from build123d import *

# Parameters (mm, degrees)
SKETCH1_R           = 10
BOSS_EXTRUDE1_DEPTH = 75
SKETCH2_R           = 9.5
CUT_EXTRUDE1_DEPTH  = 77.321687612
SKETCH4_W           = 0.5
SKETCH4_H           = 10


with BuildPart() as part:
    # Sketch1 → Boss-Extrude1 (new body)
    with BuildSketch(Plane(origin=(0, 0, 0), x_dir=(1, 0, 0), z_dir=(0, 1, 0))):
        with Locations(Location((0, 0, 0), (0, 0, 270))):
            Circle(SKETCH1_R)
    extrude(amount=BOSS_EXTRUDE1_DEPTH)

    # Sketch2 → Cut-Extrude1 (cut, through all)
    with BuildSketch(Plane(origin=(0, 75, 0), x_dir=(1, 0, 0), z_dir=(0, 1, 0))):
        with Locations(Location((0, 0, 0), (0, 0, 270))):
            Circle(SKETCH2_R)
    extrude(amount=-CUT_EXTRUDE1_DEPTH, mode=Mode.SUBTRACT)

    # Sketch3 → Revolve1 (revolve)
    with BuildSketch(Plane(origin=(0, 0, 0), x_dir=(0, 0, -1), z_dir=(1, 0, 0)), mode=Mode.PRIVATE) as revolve1_sk:
        Polygon((10, 75), (12.75, 85), (12.25, 85), (9.5, 75), align=None)
    revolve(revolve1_sk.sketch.rotate(Axis((0, 75, 0), (0, -1, 0)), 180), axis=Axis((0, 75, 0), (0, -1, 0)))

    # Sketch4 → Revolve2 (revolve)
    with BuildSketch(Plane(origin=(0, 0, 0), x_dir=(0, 0, -1), z_dir=(1, 0, 0)), mode=Mode.PRIVATE) as revolve2_sk:
        with Locations((12.5, 90)):
            Rectangle(SKETCH4_W, SKETCH4_H)
    revolve(revolve2_sk.sketch.rotate(Axis((0, 75, 0), (0, -1, 0)), 180), axis=Axis((0, 75, 0), (0, -1, 0)))


solid = part.part
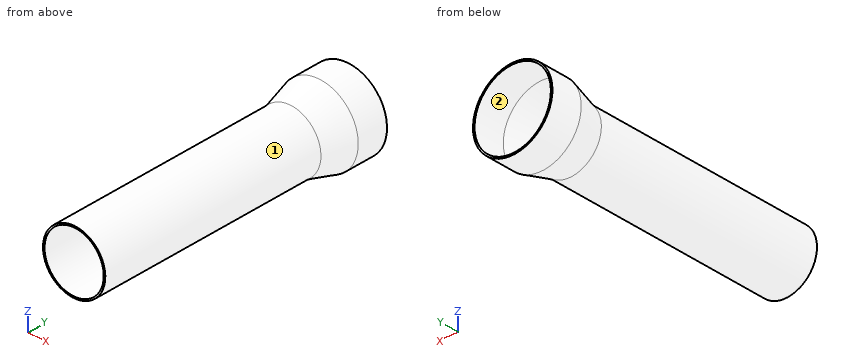
Can you work these out from the model? Positions are in its coordinate system, mm. Face numbers are marked on the shaded views. Give positions to 0.01 mm unless a question says otherwise; leave off trailing zeros. Order: outer loops, then holes, each group sorted by start corner. A loop starts at its lowest first (then second) coordinate and runs counter-clockwise, first axis right, second up. Notation, with made-up numbers: M 53,25 L 84,25 A27 cw 84,57 Z; hole C 36,42.25 d8. An arc over 180 degrees is marked long. Use a Markdown table: item, result. Add a question column.
Item 1: Suppose I cut it at D-D (y = 29). List the corners of the cut face in (x, z) for me, then the cut area to 3 significant figures.
Item 2: Suppose I cut it at B-B (z = 0). List the corners of the cut face in (x, y) for me, then the cut area to 3 significant figures.
Item 3: Will these pins go through, and if not, where does the flat tip stop? pin 1 (8 mm diameter, centred on x = -9, y = 18.5, fed in from -Z); pin 2 (4 mm diameter, centred on x = 5, y = 14, fed in from -Z); pin 3 (1 mm diameter, centred on x = 3.5, z = -7, fed in from -Y); pin 4 (1.5 mm diameter, centred on x = 0, y = 31.5, fed in from +Z).
Item 4: Suppose I cut it at C-C (y = 87). List the corners of the cut face in (x, z) for me.
Item 5: Suppose I cut it at A-A (x = 0). List the corners of the cut face in (y, z) for me.
Item 6: If I drill on L1, parallel to X at y = 32, z = 0; L2, parallel to X at y = 90.25, z = 0; L3, parallel to Z at x = -0.5, y = 73, over which ranges is the centre line in solid material (lowest first)? Write a range as [from, to].
Item 7: We'd pull the mould along Z, two halves only. Please class the marked faces 1 and 2: +Z half, -Z half, draft (parallel to the pull), parting line (faces both ways), or undercut.
Answer sheet:
| question | item | result |
|---|---|---|
| 1 | outline | C 0,0 d20; hole C 0,0 d19 |
| 1 | area | 30.6 mm² |
| 2 | outline | M -12.75,85 L -10,75 L -10,0 L -9.5,0 L -9.5,75 L -12.25,85 L -12.25,95 L -12.75,95 Z; M 9.5,0 L 10,0 L 10,75 L 12.75,85 L 12.75,95 L 12.25,95 L 12.25,85 L 9.5,75 Z |
| 2 | area | 95.0 mm² |
| 3 | pin 1 | stops at z = -8.66 |
| 3 | pin 2 | stops at z = -9.54 |
| 3 | pin 3 | passes through |
| 3 | pin 4 | stops at z = 10 |
| 4 | outline | C 0,0 d25.5; hole C 0,0 d24.5 |
| 5 | outline | M 0,-10 L 75,-10 L 85,-12.75 L 95,-12.75 L 95,-12.25 L 85,-12.25 L 75,-9.5 L 0,-9.5 Z; M 0,9.5 L 75,9.5 L 85,12.25 L 95,12.25 L 95,12.75 L 85,12.75 L 75,10 L 0,10 Z |
| 6 | L1 | x = [-10, -9.5], [9.5, 10] |
| 6 | L2 | x = [-12.75, -12.25], [12.25, 12.75] |
| 6 | L3 | z = [-9.99, -9.49], [9.49, 9.99] |
| 7 | face 1 | parting line |
| 7 | face 2 | undercut |
